Autodesk Inventor part; units mm, degrees
ref_plane "YZ Plane" through (0, 0, 0) normal (1, 0, 0) x (0, 1, 0)
ref_plane "XZ Plane" through (0, 0, 0) normal (0, 1, 0) x (-1, 0, 0)
ref_plane "XY Plane" through (0, 0, 0) normal (0, 0, 1) x (1, 0, 0)
sketch "Sketch1" plane through (0, 0, 0) normal (0, 0, 1) x (1, 0, 0)
  line L0 (-13, 12) -> (13, 12)
  line L1 (13, 12) -> (13, -12)
  line L2 (13, -12) -> (-13, -12)
  line L3 (-13, -12) -> (-13, 12)
  line L4 (-13, 3.25) -> (-15, 3.25)
  line L5 (-15, 3.25) -> (-15, -3.25)
  line L6 (-15, -3.25) -> (-13, -3.25)
  line L7 (-13, -3.25) -> (-13, 3.25)
  line L8 (13, 3.25) -> (15, 3.25)
  line L9 (15, 3.25) -> (15, -3.25)
  line L10 (15, -3.25) -> (13, -3.25)
  line L11 (13, -3.25) -> (13, 3.25)
  line L12 (-25.4, 25.4) -> (25.4, 25.4)
  line L13 (25.4, 25.4) -> (25.4, -25.4)
  line L14 (25.4, -25.4) -> (-25.4, -25.4)
  line L15 (-25.4, -25.4) -> (-25.4, 25.4)
  circle A0 centre (0, 0) radius 7.1437
  circle A1 centre (-3, 12) radius 1.5
  line L16 (-13, 8) -> (-9, 12)
  line L17 (9, 12) -> (13, 8)
  line L18 (13, -8) -> (9, -12)
  line L19 (-13, -8) -> (-9, -12)
  point P0 (-14, 3.25)
  point P1 (14, 3.25)
  point P2 (-14, -3.25)
  point P3 (14, -3.25)
  point P4 (-20.32, 20.32)
  point P5 (20.32, 20.32)
  point P6 (20.32, -20.32)
  point P7 (-20.32, -20.32)
  dimension "d0" = 24
  dimension "d1" = 12
  dimension "d2" = 26
  dimension "d3" = 13
  dimension "d4" = 2
  dimension "d5" = 6.5
  dimension "d6" = 3.25
  dimension "d7" = 2
  dimension "d8" = 14.2875
  dimension "d9" = 50.8
  dimension "d10" = 25.4
  dimension "d11" = 50.8
  dimension "d12" = 25.4
  dimension "d13" = 3
  dimension "d14" = 10
  dimension "d15" = 4
  dimension "d16" = 4
  dimension "d17" = 4
  dimension "d18" = 4
  dimension "d19" = 4
  dimension "d20" = 5.08
  dimension "d21" = 5.08
  dimension "d22" = 5.08
  dimension "d23" = 5.08
  dimension "d34" = 40.64
  dimension "d35" = 40.64
extrude "Extrusion1" add sketch "Sketch1" against normal blind 3.175 contours L0 L16 L3 | L0 L1 L17 | L19 L2 L3 | L18 L1 L2 | L12 L13 L14 L15
fillet "Fillet1" radius 3.175 4 edges at (-13, -3.25, -1.5875) (-13, 3.25, -1.5875) (13, 3.25, -1.5875) (13, -3.25, -1.5875)
hole "Hole1" at (-20.32, 20.32, 0) at (20.32, 20.32, 0) at (20.32, -20.32, 0) at (-20.32, -20.32, 0) direction (0, 0, -1) diameter 4.572 end through all
thread "Thread1"
thread "Thread2"
thread "Thread3"
thread "Thread4"
fillet "Fillet2" radius 4.7625 4 edges at (25.4, 25.4, -1.5875) (25.4, -25.4, -1.5875) (-25.4, 25.4, -1.5875) (-25.4, -25.4, -1.5875)
equation "\"d7\" = d4"
equation "\"d16\" = d15"
equation "\"d17\" = d15"
equation "\"d18\" = d15"
equation "\"d19\" = d15"
properties part number "BD gearbox mount block"
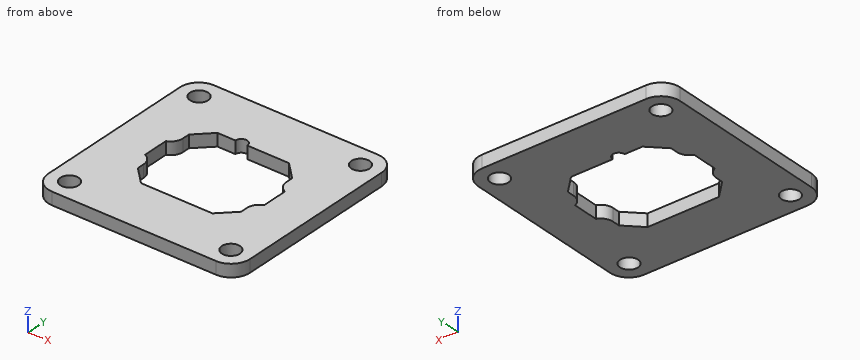
Input: part model. Units: mm. Frame: model coordinates. Give positions to 0.01 mm unless a question says otherwise; leave off trailing zeros. Loops run counter-clockwise (first coordinate to the right, second up) from the corner with the lowest first, then second, coordinate; pieces in that order, holes last. Notation, with made-up numbers: M -27.75,-17 L -20.75,-17 A12 ccw -20.75,-12 Z; hole C 2,28.5 d11. An arc over 180 degrees is marked long. Use one line per item in the form item = value.
1. Section query A-A, the plane x = 2.5. Return the cut outline in (y, z) (3 decimals), and give its area (3 significant figures).
Numbers:
outline = M -25.4,-3.175 L -12,-3.175 L -12,0 L -25.4,0 Z; M 12,-3.175 L 25.4,-3.175 L 25.4,0 L 12,0 Z
area = 85.1 mm²
2. Section query B-B, the plane y = 10.5. Return the cut outline in (x, z) (3 decimals), and give its area (3 significant figures).
Numbers:
outline = M -25.4,-3.175 L -10.5,-3.175 L -10.5,0 L -25.4,0 Z; M 10.5,-3.175 L 25.4,-3.175 L 25.4,0 L 10.5,0 Z
area = 94.6 mm²
3. Section query C-C, the plane z = -0.6. Count the separate pieces of the cut face and the enclosed holes in it, and give its area (3 significant figures).
Numbers:
separate_pieces = 1
enclosed_holes = 5
area = 1,870 mm²
4. Line query: L1, parallel to Y at x = -20.5, z = -2.5; L2, parallel to X at y = 20.32, z = -2.35; L3, parallel to Y at x = -22, z = -1.25. Output: solid intervals per line, ascending.
Numbers:
L1 = -25.4 to -22.6, -18.04 to 18.04, 22.6 to 25.4
L2 = -25.4 to -22.61, -18.03 to 18.03, 22.61 to 25.4
L3 = -25.2 to -21.87, -18.77 to 18.77, 21.87 to 25.2
5. Section query D-D, the plane y = -19.5. Return the cut outline in (x, z) (3 decimals).
Numbers:
outline = M -25.4,-3.175 L -22.454,-3.175 L -22.454,0 L -25.4,0 Z; M -18.186,-3.175 L 18.186,-3.175 L 18.186,0 L -18.186,0 Z; M 22.454,-3.175 L 25.4,-3.175 L 25.4,0 L 22.454,0 Z
